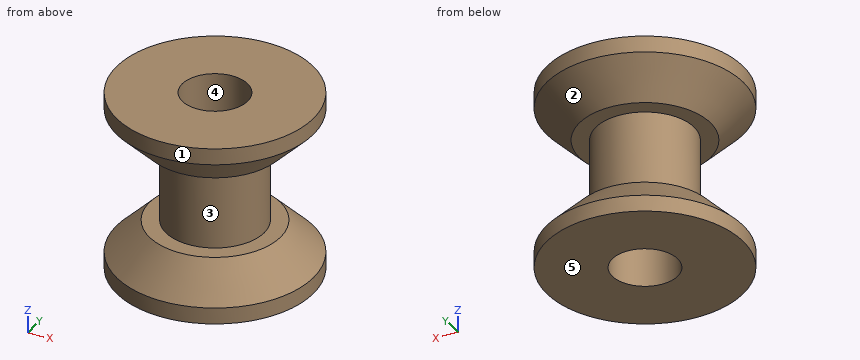
```python
from build123d import *

# Parameters (mm, degrees)
F0_R     = 7.62
F1_DEPTH = 3.81
F2_R     = 3.81
F3_DEPTH = 6.35
F4_R     = 7.62
F5_DEPTH = 3.81
F7_D     = 5.08
F8_SIZE  = 2.54


with BuildPart() as f1:
    # F0 (on Top) → F1 (new body)
    with BuildSketch(Plane.XY):
        with Locations((-5.842393, 4.891916)):
            Circle(F0_R)
    extrude(amount=F1_DEPTH)

    # F2 (on face) → F3 (join)
    with BuildSketch(Plane.XY.offset(3.81)):
        with Locations((-5.842393, 4.891916)):
            Circle(F2_R)
    extrude(amount=F3_DEPTH)

    # F4 (on face) → F5 (join)
    with BuildSketch(Plane.XY.offset(10.16)):
        with Locations((-5.842393, 4.891916)):
            Circle(F4_R)
    extrude(amount=F5_DEPTH)

    # F7 (through all)
    with Locations(Plane.XY.offset(13.97)):
        with Locations((-5.842393, 4.891916)):
            Hole(F7_D / 2)

    # F8
    f8_edges = [f1.edges().sort_by_distance(p)[0] for p in [
        (-13.462393, 4.891916, 10.16),
        (-13.462393, 4.891916, 3.81),
    ]]
    chamfer(f8_edges, length=F8_SIZE)


solid = f1.part
```
CAD build for the part. Positions are in the model's coordinates, mm. Face numbers are marked on the shaded views. A direction names the side the tool comes from. Coordinates: 2 decimals unless noted, no trailing zeros. Order: outer loops, then holes, each group sorted by start corner. A loop starts at its lowest first (then second) coordinate and runs counter-clockwise, first axis right, second up.
(1) Saw through at A-A, the plane z = 3. Write the cut outline in (x, y).
Solution:
outline: circle Ø11.78 at (-5.84, 4.89); hole circle Ø5.08 at (-5.84, 4.89)
(2) Saw through at B-B, the plane z = 5.75. Write the cut outline in (x, y), and give its area (3 significant figures).
Solution:
outline: circle Ø7.62 at (-5.84, 4.89); hole circle Ø5.08 at (-5.84, 4.89)
area: 25.3 mm2
(3) Drill centre lines: L1, parallel to Z at x = -4.5, y = 9.75; L2, parallel to Y at x = -6, z = 6; L3, parallel to Y at x = -4.25, z = 13.25. Where is each one in solid material? Low to high.
Solution:
L1: z = 0 to 3.81, 10.16 to 13.97
L2: y = 1.09 to 2.36, 7.43 to 8.7
L3: y = -2.56 to 2.91, 6.87 to 12.34
(4) Which spindle directions (+Z, -Z, +X, -X, +Y, -Y) get a long thin tool onto all of the face, cutting with end or side? Do the marked faces 1 and 2. Say none if no direction does.
Solution:
face 1: +Z, -Z
face 2: none
(5) Pin check, flat tips, straight feed: pin 1 Ø6 at (y, z) = (6, 9) entering from -X; pin 2 Ø1 at (x, y) = (-5.5, 6) entering from -Z; pin 3 Ø6 at (y, z) = (0.5, 3.5) entering from +X; pin 4 Ø2 at (x, z) = (-1.5, 6.5) entering from -Y. Stop position of each tip, or through.
Solution:
pin 1: stops at x = -12.7
pin 2: passes through
pin 3: stops at x = 1.39
pin 4: stops at y = 3.06
(6) Mould opens along X. For the marked faces 3, 4 and 5 say: released by +X, released by -X, zero draft, split by the parting line, or undercut.
Solution:
face 3: split by the parting line
face 4: undercut
face 5: zero draft
